from build123d import *

# Parameters (mm, degrees)
SKETCH1_W           = 105
SKETCH1_H           = 12.7
SKETCH1_R           = 2.5
BOSS_EXTRUDE1_DEPTH = 3.175
SKETCH2_W           = 3.175
SKETCH2_H           = 12.7
BOSS_EXTRUDE2_DEPTH = 90
SKETCH3_R           = 3
CUT_EXTRUDE1_DEPTH  = 3.175
FILLET1_R           = 5
FILLET2_R           = 7


with BuildPart() as part:
    # Sketch1 → Boss-Extrude1 (new body)
    with BuildSketch(Plane(origin=(0, 0, 0), x_dir=(1, 0, 0), z_dir=(0, 1, 0))):
        Rectangle(SKETCH1_W, SKETCH1_H)
        with Locations(Location((42.5, 0, 0), (0, 0, 270))):
            Circle(SKETCH1_R, mode=Mode.SUBTRACT)
        with Locations(Location((-7.5, 0, 0), (0, 0, 270))):
            Circle(SKETCH1_R, mode=Mode.SUBTRACT)
    extrude(amount=BOSS_EXTRUDE1_DEPTH)

    # Sketch2 → Boss-Extrude2 (add)
    with BuildSketch(Plane(origin=(0, 3.175, 0), x_dir=(1, 0, 0), z_dir=(0, 1, 0))):
        with Locations((-50.9125, 0)):
            Rectangle(SKETCH2_W, SKETCH2_H)
    extrude(amount=BOSS_EXTRUDE2_DEPTH)

    # Sketch3 → Cut-Extrude1 (cut)
    with BuildSketch(Plane.ZY.offset(52.5)):
        with Locations((0, 56.51)):
            Circle(SKETCH3_R)
        with Locations((0, 81.656)):
            Circle(SKETCH3_R)
    extrude(amount=-CUT_EXTRUDE1_DEPTH, mode=Mode.SUBTRACT)

    # Fillet1
    fillet1_edges = [part.edges().sort_by_distance(p)[0] for p in [
        (-49.325, 3.175, 0),
    ]]
    fillet(fillet1_edges, radius=FILLET1_R)

    # Fillet2
    fillet2_edges = [part.edges().sort_by_distance(p)[0] for p in [
        (-52.5, 0, 0),
    ]]
    fillet(fillet2_edges, radius=FILLET2_R)


solid = part.part
The listing builds one solid part. Answer for the finished solid, in the listing's coordinates (mm). A direction names the side the tool comes from. Give positions to 0.01 mm unless a question says otherwise; leave off trailing zeros. Write each loop counter-clockwise with the first axis right and the second up, starting at its lowest first coordinate (ties: lowest second). Pieces come first, ordered by that corner, then holes. Notation, with made-up numbers: (-2.75, 13.5) -> (32.25, 13.5) arc R10 cw to (32.25, 19.5) -> close; hole circle Ø1 at (74, -3). An arc over 180 degrees is marked (long way). One line per question, with ' | ' between items. Start each with the question number.
1. Find the intervals of material crossed by probe 1 along Y at (x, z) = (-50.6, 0) (3 decimals); probe 2 along Y at (x, z) = (-51.2, 0) (3 decimals); probe 3 along X at (y, z) = (62, 3.5) (3 decimals), in increasing order.
2. For a pull along Y with two mould halves and no side action, classify faces 3 (the cylindrical face through (-50.93, 53.58, -0.65)), 4 (the flat face through (52.5, 2, 0)), 5 (the cylindrical face through (-50.93, 84.63, -0.39)), 6 (the flat face through (-51, 93.175, 0)) as pulls with the +Y half, pulls with the -Y half, needs draft (parallel to the pull), parting line crosses it, or undercut.
3. Section D-D (y = 43) is taken. Determine the outline of the cut face in (x, z) (3 decimals), plus the area to 3 significant figures.
4. Section B-B (y = 56.51) is taken. Determine the outline of the cut face in (x, z) (3 decimals), plus the area to 3 significant figures.
5. Section C-C (x = 42.5) is taken. Determine the outline of the cut face in (y, z) (3 decimals), plus the area to 3 significant figures.
6. For faces 1 (the cylindrical face through (40.06, 1.57, -0.54)), 2 (the flat face through (-49.325, 50, 0)), determine the directions among +Z, -Z, +X, -X, +Y, -Y from which every point of the face is accessible in a straight line to the end or side of a thin tool.
7. Section A-A (z = 0) is taken. Determine the outline of the cut face in (x, y) (3 decimals).
Response values:
1) probe 1: 2.205 to 53.51, 59.51 to 78.656, 84.656 to 93.175 | probe 2: 2.937 to 53.51, 59.51 to 78.656, 84.656 to 93.175 | probe 3: -52.5 to -49.325
2) face 3: undercut | face 4: needs draft | face 5: undercut | face 6: pulls with the +Y half
3) outline: (-52.5, -6.35) -> (-49.325, -6.35) -> (-49.325, 6.35) -> (-52.5, 6.35) -> close | area: 40.3 mm2
4) outline: (-52.5, -6.35) -> (-49.325, -6.35) -> (-49.325, -3) -> (-52.5, -3) -> close; (-52.5, 3) -> (-49.325, 3) -> (-49.325, 6.35) -> (-52.5, 6.35) -> close | area: 21.3 mm2
5) outline: (0, -6.35) -> (3.175, -6.35) -> (3.175, -2.5) -> (0, -2.5) -> close; (0, 2.5) -> (3.175, 2.5) -> (3.175, 6.35) -> (0, 6.35) -> close | area: 24.4 mm2
6) face 1: +Y, -Y | face 2: +Z, -Z, +X, +Y
7) outline: (-52.5, 7) arc R7 ccw to (-45.5, 0) -> (-10, 0) -> (-10, 3.175) -> (-44.325, 3.175) arc R5 cw to (-49.325, 8.175) -> (-49.325, 53.51) -> (-52.5, 53.51) -> close; (-52.5, 59.51) -> (-49.325, 59.51) -> (-49.325, 78.656) -> (-52.5, 78.656) -> close; (-52.5, 84.656) -> (-49.325, 84.656) -> (-49.325, 93.175) -> (-52.5, 93.175) -> close; (-5, 0) -> (40, 0) -> (40, 3.175) -> (-5, 3.175) -> close; (45, 0) -> (52.5, 0) -> (52.5, 3.175) -> (45, 3.175) -> close
